from build123d import *

# Parameters (mm, degrees)
F1_DEPTH = 15
F2_R     = 2


with BuildPart() as f1:
    # F0 (on Top) → F1 (new body)
    with BuildSketch(Plane.XY):
        with BuildLine():
            Line((0, 49.473686), (-30, 49.473686))
            Line((-30, 49.473686), (-30, 39.473686))
            Line((-30, 39.473686), (-20, 39.473686))
            Line((-20, 39.473686), (-20, 19.473686))
            Line((-20, 19.473686), (-30, 19.473686))
            ThreePointArc((-30, 19.473686), (-20, 9.473686), (-10, 19.473686))
            Line((-10, 19.473686), (-10, 39.473686))
            Line((-10, 39.473686), (0, 39.473686))
            Line((0, 39.473686), (0, 49.473686))
        make_face()
    extrude(amount=F1_DEPTH)

    # F2
    f2_edges = [f1.edges().sort_by_distance(p)[0] for p in [
        (-25, 39.473686, 15),
        (-30, 44.473686, 15),
        (-15, 49.473686, 15),
        (0, 44.473686, 15),
        (-5, 39.473686, 15),
        (-10, 29.473686, 15),
        (-20, 9.473686, 15),
        (-25, 19.473686, 15),
        (-20, 29.473686, 15),
        (-10, 39.473686, 7.5),
        (0, 39.473686, 7.5),
        (0, 49.473686, 7.5),
        (-30, 39.473686, 7.5),
        (-30, 49.473686, 7.5),
        (-30, 19.473686, 7.5),
        (-20, 19.473686, 7.5),
        (-25, 19.473686, 0),
        (-25, 39.473686, 0),
        (-15, 49.473686, 0),
        (-30, 44.473686, 0),
        (-20, 9.473686, 0),
        (-20, 29.473686, 0),
        (-10, 29.473686, 0),
        (-5, 39.473686, 0),
        (0, 44.473686, 0),
        (-20, 39.473686, 7.5),
    ]]
    fillet(f2_edges, radius=F2_R)


solid = f1.part
Could you check a few things on this model? Use its own coordinates, in mm. A direction names the side the tool comes from. Coordinates: 2 decimals unless noted, no trailing zeros. Loops run counter-clockwise (first coordinate to the right, second up) from the corner with the lowest first, then second, coordinate; pieces in that order, holes last. Notation, with made-up numbers: (34, -7.75) -> (39, -7.75) arc R19 cw to (39, 22.25) -> close; hole circle Ø6 at (31.5, 78.5). An arc over 180 degrees is marked (long way). Answer in a Markdown table with one row per item.
(1) Imagine slicing it at A-A (y = 25.5). List the corners of the cut face in (x, z) for me, plus the area to 3 significant figures.
Results found:
| item | result |
|---|---|
| outline | (-20, 2) arc R2 ccw to (-18, 0) -> (-12, 0) arc R2 ccw to (-10, 2) -> (-10, 13) arc R2 ccw to (-12, 15) -> (-18, 15) arc R2 ccw to (-20, 13) -> close |
| area | 147 mm^2 |
(2) Imagine slicing it at C-C (z = 8). List the corners of the cut face in (x, y) for me, plus the area to 3 significant figures.
Results found:
| item | result |
|---|---|
| outline | (-30, 41.47) arc R2 ccw to (-28, 39.47) -> (-22, 39.47) arc R2 cw to (-20, 37.47) -> (-20, 21.47) arc R2 cw to (-22, 19.47) -> (-27.75, 19.47) arc R2 ccw to (-29.68, 16.97) arc R10 ccw to (-10, 19.47) -> (-10, 37.47) arc R2 cw to (-8, 39.47) -> (-2, 39.47) arc R2 ccw to (0, 41.47) -> (0, 47.47) arc R2 ccw to (-2, 49.47) -> (-28, 49.47) arc R2 ccw to (-30, 47.47) -> close |
| area | 655 mm^2 |
(3) Imagine slicing it at B-B (x = -3.5). List the corners of the cut face in (y, z) for me, plus the area to 3 significant figures.
Results found:
| item | result |
|---|---|
| outline | (39.47, 2) arc R2 ccw to (41.47, 0) -> (47.47, 0) arc R2 ccw to (49.47, 2) -> (49.47, 13) arc R2 ccw to (47.47, 15) -> (41.47, 15) arc R2 ccw to (39.47, 13) -> close |
| area | 147 mm^2 |
(4) Thinking about a two-plate mould opening in Y: for faces 6 (the face through (-24.958, 40.044, 14.399)), 7 (the face through (-29.43, 44.43, 0.6)), 8 (the face through (-4.958, 40.044, 0.601)), which applies, released by +Y, released by -Y, zero draft, split by the parting line, or undercut?
Results found:
| item | result |
|---|---|
| face 6 | undercut |
| face 7 | zero draft |
| face 8 | released by -Y |
(5) If I drill on probe 1 along X at (y, z) = (21.5, 8.75); probe 2 along Y at (x, z) = (-2.5, 4); probe 3 along Y at (x, z) = (-26.5, 13.25) (3 decimals), over which ranges is the centre line in solid material (lowest first)?
Results found:
| item | result |
|---|---|
| probe 1 | x = -20 to -10 |
| probe 2 | y = 39.47 to 49.47 |
| probe 3 | y = 11.895 to 19.458, 39.489 to 49.458 |
(6) For faces 1 (the face through (-19.43, 29.36, 0.6)), 2 (the face through (-4.958, 40.044, 14.399)), 3 (the face through (-24.9, 18.9, 14.4)), 4 (the face through (-25, 39.474, 7)), 5 (the face through (-10.57, 28.6, 0.6)), which set-ups out of +Z, -Z, +X, -X, +Y, -Y let a thin tool reach every point of the face, with its end or its side?
Results found:
| item | result |
|---|---|
| face 1 | -Z, -X |
| face 2 | +Z, +X, -Y |
| face 3 | +Z, -X |
| face 4 | +Z, -Z, -X |
| face 5 | -Z, +X, -Y |
(7) Will these pins go through, and if not, where does the flat tip stop? pin 1 Ø6.5 at (x, z) = (-5, 6.5) entering from -Y; pin 2 Ø1.5 at (y, z) = (39, 12) entering from +X; pin 3 Ø3.5 at (y, z) = (28, 5) entering from -X; pin 4 Ø1 at (x, y) = (-23.5, 16) entering from -Z.
Results found:
| item | result |
|---|---|
| pin 1 | stops at y = 39.46 |
| pin 2 | stops at x = -0.99 |
| pin 3 | stops at x = -20 |
| pin 4 | stops at z = 0 |
